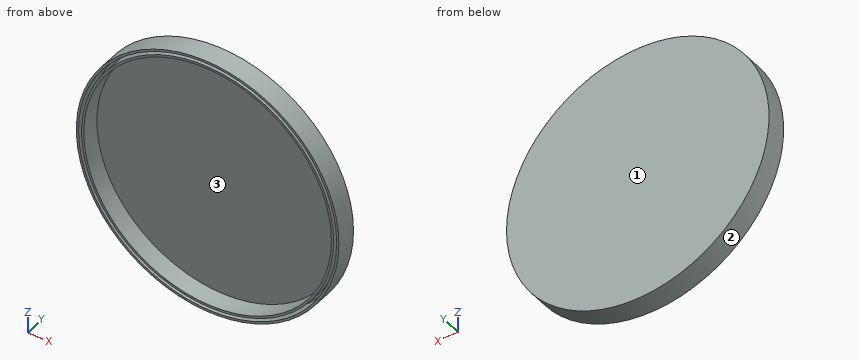
```python
from build123d import *

# Parameters (mm, degrees)
F0_R     = 35.1
F0_R_2   = 34.5
F1_DEPTH = 5
F0_R_3   = 33.6999967694
F0_R_4   = 33.0999977887
F2_DEPTH = 0.6


with BuildPart() as f1:
    # F0 (on Front) → F1 (new body)
    with BuildSketch(Plane.XZ):
        Circle(F0_R)
        Circle(F0_R_2, mode=Mode.SUBTRACT)
    extrude(amount=F1_DEPTH)



with BuildPart() as f1b:
    # F0 (on Front) → F1, piece 2 (new body)
    with BuildSketch(Plane.XZ):
        Circle(F0_R_3)
        Circle(F0_R_4, mode=Mode.SUBTRACT)
    extrude(amount=F1_DEPTH)


with BuildPart() as f1_1:
    add(f1.part)

    add(f1b.part)  # F2 merges F1b
    # F0 (on Front) → F2 (join)
    with BuildSketch(Plane.XZ):
        Circle(F0_R)
        Circle(F0_R_2, mode=Mode.SUBTRACT)
        Circle(F0_R_2)
        Circle(F0_R_3, mode=Mode.SUBTRACT)
        Circle(F0_R_3)
        Circle(F0_R_4, mode=Mode.SUBTRACT)
        Circle(F0_R_4)
    extrude(amount=-F2_DEPTH)


solid = f1_1.part
```
Model file for the job. Use its own axes, mm. Face numbers are marked on the shaded views. Give positions to 0.01 mm unless a question says otherwise; leave off trailing zeros. Write each loop counter-clockwise with the first axis right and the second up, starting at its lowest first coordinate (ties: lowest second). Pieces come first, ordered by that corner, then holes. Notation, with made-up numbers: (15, -18.75) -> (26, -18.75) arc R19 ccw to (26, 4.25) -> close; hole circle Ø4 at (69, -34.5). An arc over 180 degrees is marked (long way). Use CSV: the item, a comma, the result in double quotes. Start each with the question number.
1) Drill centre lines: L1, parallel to Z at x = 0, y = -1.1; L2, parallel to Z at x = 4, y = -4.4; L3, parallel to X at y = -1.75, z = -14. Where is each one in solid material? Low to high.
2) Two-plate mould, pull along X, no slides. Class the marked faces 1, 2 and 3: released by +X, released by -X, zero draft, split by the parting line, or undercut.
3) Cut at C-C on z = 0. List the corners of the cut face in (x, y).
4) Cut at B-B on x = 0. List the corners of the cut face in (y, z), plus the area to 3 significant figures.
5) Pin check, flat tips, straight feed: P1, Ø20.5, axis at x = 0.5, z = -17, coming from the -Y side; P2, Ø1.5, axis at x = 20, y = -3, coming from the +Z side; P3, Ø1.5, axis at y = -3.5, z = -10, coming from the +X side. Stop position of each tip, or through.
6) Cut at A-A on y = -1. List the corners of the cut face in (x, z), plus the area to 3 significant figures.
Final values:
1,L1,"z = -35.1 to -34.5, -33.7 to -33.1, 33.1 to 33.7, 34.5 to 35.1"
1,L2,"z = -34.87 to -34.27, -33.46 to -32.86, 32.86 to 33.46, 34.27 to 34.87"
1,L3,"x = -32.19 to -31.53, -30.65 to -29.99, 29.99 to 30.65, 31.53 to 32.19"
2,face 1,"zero draft"
2,face 2,"split by the parting line"
2,face 3,"undercut"
3,outline,"(-35.1, -5) -> (-34.5, -5) -> (-34.5, 0) -> (-33.7, 0) -> (-33.7, -5) -> (-33.1, -5) -> (-33.1, 0) -> (33.1, 0) -> (33.1, -5) -> (33.7, -5) -> (33.7, 0) -> (34.5, 0) -> (34.5, -5) -> (35.1, -5) -> (35.1, 0.6) -> (-35.1, 0.6) -> close"
4,outline,"(-5, -35.1) -> (0.6, -35.1) -> (0.6, 35.1) -> (-5, 35.1) -> (-5, 34.5) -> (0, 34.5) -> (0, 33.7) -> (-5, 33.7) -> (-5, 33.1) -> (0, 33.1) -> (0, -33.1) -> (-5, -33.1) -> (-5, -33.7) -> (0, -33.7) -> (0, -34.5) -> (-5, -34.5) -> close"
4,area,"54.1 mm2"
5,P1,"stops at y = 0"
5,P2,"stops at z = 29.35"
5,P3,"stops at x = 33.86"
6,outline,"circle Ø70.2 at (0, 0); circle Ø67.4 at (0, 0); hole circle Ø69 at (0, 0); hole circle Ø66.2 at (0, 0)"
6,area,"257 mm2"
